The listing builds one solid part. Answer for the finished solid, in the listing's coordinates (mm). A direction names the side the tool comes from. Coordinates: 2 decimals unless noted, no trailing zeros. Order: outer loops, then holes, each group sorted by start corner. A loop starts at its lowest first (then second) coordinate and runs counter-clockwise, first axis right, second up. Notation, with made-up numbers: (87.5, 73.5) - (102.5, 73.5) arc R7 cw to (102.5, 77.5) - close; hole circle Ø11 at (85.5, -18). An arc over 180 degrees is marked (long way). One line per item, written item: value. Start each with the question number.
Solid Edge part; units mm, degrees
sketch "Sketch1" plane through (0, 0, 0) normal (0, 0, 1) x (1, 0, 0)
  circle A0 centre (0, 0) radius 1.9
extrude "Protrusion1" add sketch "Sketch1" along normal blind 2
sketch "Sketch2" plane through (0, 0, 2) normal (0, 0, 1) x (0, 1, 0)
  line L0 (0, 0.866) -> (0.75, 0.433)
  line L1 (0.75, 0.433) -> (0.75, -0.433)
  line L2 (0.75, -0.433) -> (0, -0.866)
  line L3 (0, -0.866) -> (-0.75, -0.433)
  line L4 (-0.75, -0.433) -> (-0.75, 0.433)
  line L5 (-0.75, 0.433) -> (0, 0.866)
extrude "Cutout1" cut sketch "Sketch2" against normal blind 1
fillet "Round1" radius 0.2 1 edges at (-1.9, 0, 2)
sketch "Sketch3" plane through (0, 0, 0) normal (1, 0, 0) x (0, 1, 0)
  line L0 (-0.7545, -6) -> (0, -6)
  line L1 (-1, -5.7545) -> (-0.7545, -6)
  line L2 (-1, -1.2) -> (-1, -5.7545)
  line L3 (-0.7545, -1.2) -> (-1, -1.2)
  line L4 (-0.7545, -1.19) -> (-0.7545, -1.2)
  line L5 (-1, -1.19) -> (-0.7545, -1.19)
  line L6 (-1, -0.1) -> (-1, -1.19)
  arc A0 (-1, -0.1) -> (-1.1, 0) centre (-1.1, -0.1) ccw
revolve "RevolvedProtrusion1" add sketch "Sketch3" angle 360 about axis through (0, 0, -60.325) along (0, 0, 1) material side at (0, -0.3772, -5.95)
cosmetic_thread "Thread1"
sketch "Sketch4" plane through (0, 0, 0) normal (0, -1, 0) x (1, 0, 0)
  line L0 (-0.865, 2) -> (0, 1.5006)
revolve "RevolvedCutout1" cut sketch "Sketch4" angle 360 about axis through (0, 0, 57.15) along (0, 0, -1) material side at (-0.4075, 0, 1.7936)
properties material "Stahl"
(1) For a pull along Y with two mould halves and no side action, classify faces 1 (the face through (0, 0, -6)), 2 (the face through (1, 0, -1)), 3 (the face through (0, -0.75, 1.5)) as pulls with the +Y half, pulls with the -Y half, needs draft (parallel to the pull), parting line crosses it, or undercut.
(2) The part is cut by section A-A on z = 1.25. Determine the outline of the cut face in (x, y).
(3) Flat-ended cylindrical pins translate along their axes: pin 1 Ø1.5 at (x, z) = (1.5, -3.5) entering from +Y; pin 2 Ø1.5 at (x, z) = (0, -1.5) entering from -Y; pin 3 Ø1.2 at (x, y) = (0, 0) entering from +Z. Find the tip coordinate at first contact, or state that the pin passes through.
(4) The part is cut by section C-C on z = -3.75. Determine the outline of the cut face in (x, y).
(5) Consider probe 1 along Y at (x, z) = (0.35, 1.75); probe 2 along Z at (x, y) = (0.1, -1.55); probe 3 along Z at (x, y) = (0, -0.55). Determine where each line is inside the solid, lowest interval first.
(6) For faces 4 (the face through (1, -1, 2)), 5 (the face through (0, 0.75, 1.5)), 6 (the face through (1, 0, -4)), determine the directions among +Z, -Z, +X, -X, +Y, -Y from which every point of the face is accessible in a straight line to the end or side of a thin tool.
Completed:
1. face 1: needs draft
1. face 2: parting line crosses it
1. face 3: undercut
2. outline: circle Ø3.8 at (0, 0); hole (-0.87, 0) - (-0.43, -0.75) - (0.43, -0.75) - (0.87, 0) - (0.43, 0.75) - (-0.43, 0.75) - close
3. pin 1: stops at y = 0.66
3. pin 2: stops at y = -1
3. pin 3: stops at z = 1
4. outline: circle Ø2 at (0, 0)
5. probe 1: y = -1.87 to -0.75, 0.75 to 1.87
5. probe 2: z = 0 to 2
5. probe 3: z = -6 to 1
6. face 4: +Z, +X, -X, +Y, -Y
6. face 5: +Z
6. face 6: -Z
